```python
from build123d import *

# Parameters (mm, degrees)
F1_DEPTH = 10
F2_R     = 12.2
F3_DEPTH = 8
F4_R     = 6
F5_DEPTH = 25
F6_R     = 1.5
F7_DEPTH = 8


with BuildPart() as f1:
    # F0 (on Front) → F1 (new body)
    with BuildSketch(Plane.XZ):
        with BuildLine():
            Line((16, 0), (-16, 0))
            ThreePointArc((-16, 0), (0, -16), (16, 0))
        make_face()
        with BuildLine():
            Line((-16, 16), (-16, 0))
            ThreePointArc((-16, 0), (-11.3137085183, 11.3137084797), (-5.46e-08, 16))
            Line((-5.46e-08, 16), (-16, 16))
        make_face()
        with BuildLine():
            ThreePointArc((-5.46e-08, 16), (-11.3137085183, 11.3137084797), (-16, 0))
            Line((-16, 0), (16, 0))
            ThreePointArc((16, 0), (11.3137084797, 11.3137085183), (-5.46e-08, 16))
        make_face()
        with BuildLine():
            ThreePointArc((-5.46e-08, 16), (11.3137084797, 11.3137085183), (16, 0))
            Line((16, 0), (16, 16))
            Line((16, 16), (-5.46e-08, 16))
        make_face()
    extrude(amount=F1_DEPTH)

    # F2 (on face) → F3 (cut)
    with BuildSketch(Plane(origin=(0, 0, 0), x_dir=(-1, 0, 0), z_dir=(0, 1, 0))):
        Circle(F2_R)
    extrude(amount=-F3_DEPTH, mode=Mode.SUBTRACT)

    # F4 (on face) → F5 (cut)
    with BuildSketch(Plane(origin=(0, -8, 0), x_dir=(-1, 0, 0), z_dir=(0, 1, 0))):
        Circle(F4_R)
    extrude(amount=-F5_DEPTH, mode=Mode.SUBTRACT)

    # F6 (on face) → F7 (cut)
    with BuildSketch(Plane.XY.offset(16)):
        with Locations((-12, -5)):
            Circle(F6_R)
        with Locations((12, -5)):
            Circle(F6_R)
    extrude(amount=-F7_DEPTH, mode=Mode.SUBTRACT)


solid = f1.part
```
Geometry: final body of the model. Coordinates: model frame, mm. A direction names the side the tool comes from. Round coordinates to 2 decimals unless told otherwise and drop trailing zeros. Order: outer loops, then holes, each group sorted by start corner. A loop starts at its lowest first (then second) coordinate and runs counter-clockwise, first axis right, second up. Notation, with made-up numbers: M 37,49.5 L 60,49.5 A16 ccw 60,58.5 Z; hole C 64,33 d3. An arc over 180 degrees is marked long. Use one line per item in the form item = value. Start each with the question number.
Q1. Material intervals for line 1 (Y direction, x = 12, z = 10.5); line 2 (Z direction, x = 0, y = -4.5); line 3 (X direction, y = -1, z = -8.5), sorted ascending. Write a range as [from, to].
Q2. Mould query, pull axis Z, two halves, no side actions, for faces 4 (the face through (-16, -5, 8)), 5 (the face through (-12, -5, 8)), 6 (the face through (-3, -8, 6)). Classes: +Z half, -Z half, draft (parallel to the pull), parting line (faces both ways), or undercut.
Q3. Access query for faces 1 (the face through (-13.5, -4.93, 12.06)), 2 (the face through (0, -5, 16)), 3 (the face through (12.19, -3.94, 0.54)). Directions: +Z, -Z, +X, -X, +Y, -Y. A direction counts if a zero-diameter tool reaches every point of the face in a straight line with its end or side. Return the directions, or none.
Q4. Cut plane D-D (z = 11.5). Return loops of the section in (x, y).
Q5. Cut plane B-B (y = -0.75). Return loops of the section in (x, z), and give its area (3 significant figures).
Q6. Cut plane C-C (z = 3). Return loops of the section in (x, y).
Q7. Pin query (flat end, axial travel): pin 1 Ø1 at (x, y) = (-11, -5) entering from -Z; pin 2 Ø1.5 at (y, z) = (-1.5, -10.5) entering from +X; pin 3 Ø1 at (y, z) = (-5, -11) entering from -X. Return the tip coordinate at first contact, or that it passes through.
Q8. Cut plane A-A (x = 0). Return loops of the section in (y, z).
Geometry results:
q1.line_1 = [-10, -6.5], [-3.5, 0]
q1.line_2 = [-16, -12.2], [12.2, 16]
q1.line_3 = [-13.56, -8.75], [8.75, 13.56]
q2.face_4 = draft
q2.face_5 = +Z half
q2.face_6 = undercut
q3.face_1 = +Z
q3.face_2 = +Z, +X, -X, +Y, -Y
q3.face_3 = +Y
q4.outline = M -16,-10 L 16,-10 L 16,0 L 4.07,0 L 4.07,-8 L -4.07,-8 L -4.07,0 L -16,0 Z; hole C -12,-5 d3; hole C 12,-5 d3
q5.outline = M -16,0 A16 ccw 16,0 L 16,16 L -16,16 Z; hole C 0,0 d24.4
q5.area = 447 mm^2
q6.outline = M -16,-10 L -5.2,-10 L -5.2,-8 L -11.83,-8 L -11.83,0 L -16,0 Z; M 5.2,-10 L 16,-10 L 16,0 L 11.83,0 L 11.83,-8 L 5.2,-8 Z
q7.pin_1 = -12.07
q7.pin_2 = 12.69
q7.pin_3 = -12.07
q8.outline = M -10,-16 L 0,-16 L 0,-12.2 L -8,-12.2 L -8,-6 L -10,-6 Z; M -10,6 L -8,6 L -8,12.2 L 0,12.2 L 0,16 L -10,16 Z
